Input: dimensioned drawing with shaded views. Units: mm. Origin: part minimum x, y, z. Round coordinates to 2 decimals unless told otherwise and drop trailing zeros. Order: outer loops, then holes, each group sorted by start corner. A loop starts at its lowest first (then second) coordinate and runs counter-clockwise, first axis right, second up.
Item 1: Mould query, pull axis X, two halves, no side actions, for the marked faces 1, 2 and 3. Classes: released by +X, released by -X, zero draft, split by the parting line, or undercut.
Item 2: Cut plane C-C on z = 16.5. Output: boundary loops of the cut face in (x, y).
Item 3: First-contact query: pin 1 (2 mm diameter, centred on x = 17.5, z = 6.5, fed in from -Y); pin 2 (4 mm diameter, centred on y = 7, z = 20.5, fed in from +X); pin 3 (1.5 mm diameter, centred on y = 3.5, z = 14.5, fed in from -X). Flat tips, straight axial feed; report the tip coordinate or a pass-through.
Item 4: Line query: L1, parallel to Y at x = 12.7, z = 17.25; L2, parallel to Y at x = 11.5, z = 12 (1 decimal); L3, parallel to X at y = 14.5, z = 19.5 (1 decimal). Output: solid intervals per line, ascending.
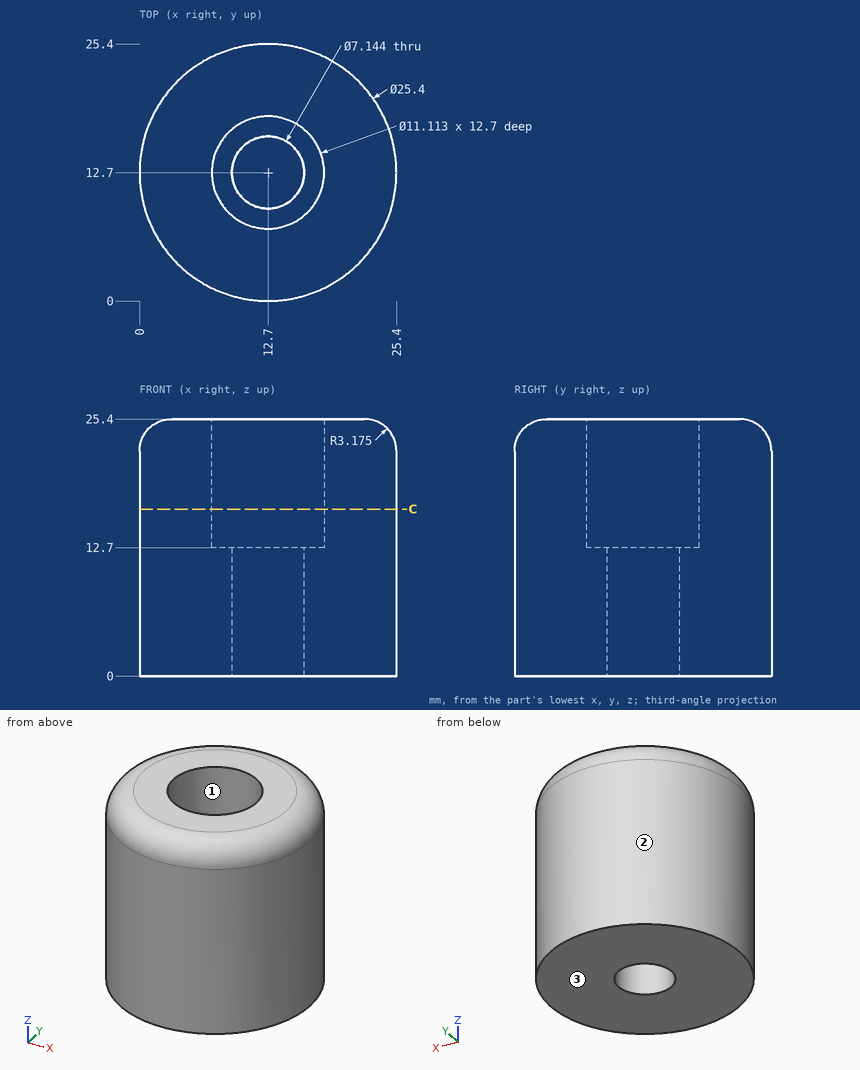
From the geometry:
1. face 1: undercut
1. face 2: split by the parting line
1. face 3: zero draft
2. outline: circle Ø25.4 at (12.7, 12.7); hole circle Ø11.11 at (12.7, 12.7)
3. pin 1: stops at y = 0.58
3. pin 2: stops at x = 24.85
3. pin 3: stops at x = 3.22
4. L1: y = 0 to 7.14, 18.26 to 25.4
4. L2: y = 0.1 to 9.3, 16.1 to 25.3
4. L3: x = 0.1 to 7.4, 18 to 25.3
